Part print with two shaded views. Sizes in mm from the minimum x, y, z corner. Give positions to 0.01 mm unless a question says otherwise; leave off trailing zeros. Write each loop counter-clockwise with the first axis right and the second up, starting at its lowest first coordinate (ties: lowest second). Pieces come first, ordered by that corner, then holes. Notation, with made-up numbers: (80, 85) - (84, 85) arc R30 ccw to (84, 108) - close; hole circle Ø1 at (-25, 62). An arc over 180 degrees is marked (long way). One line per item, written item: value. Start each with the question number.
(1) Drop flat-ended pins along their axis: P1, Ø2, axis at x = 14, z = 26, coming from the -Y side; P2, Ø1.6, axis at x = 95.5, y = 1, coming from the +Z side; P3, Ø1.2, axis at x = 96, y = 1, coming from the -Z side; P4, Ø0.8, axis at x = 7, y = 1, coming from the +Z side (1 decimal). Give the stop position or say it passes through.
(2) Probe L1, parallel to X at y = 2.95, z = 54; L2, parallel to Y at x = 19.5, z = 93.5; L3, parallel to Z at x = 11, y = 1.4 (1 decimal). List the from-to ranges inside material, lowest first.
(3) Cut at A-A, the plane x = 72.5. List the corners of the cut face in (y, z).
(4) Cut at B-B, the plane y = 2.8. List the corners of the cut face in (x, z).
(5) Mould opens along X. For the marked faces 1 and 2 say: pulls with the +X half, pulls with the -X half, needs draft (parallel to the pull), parting line crosses it, or undercut.
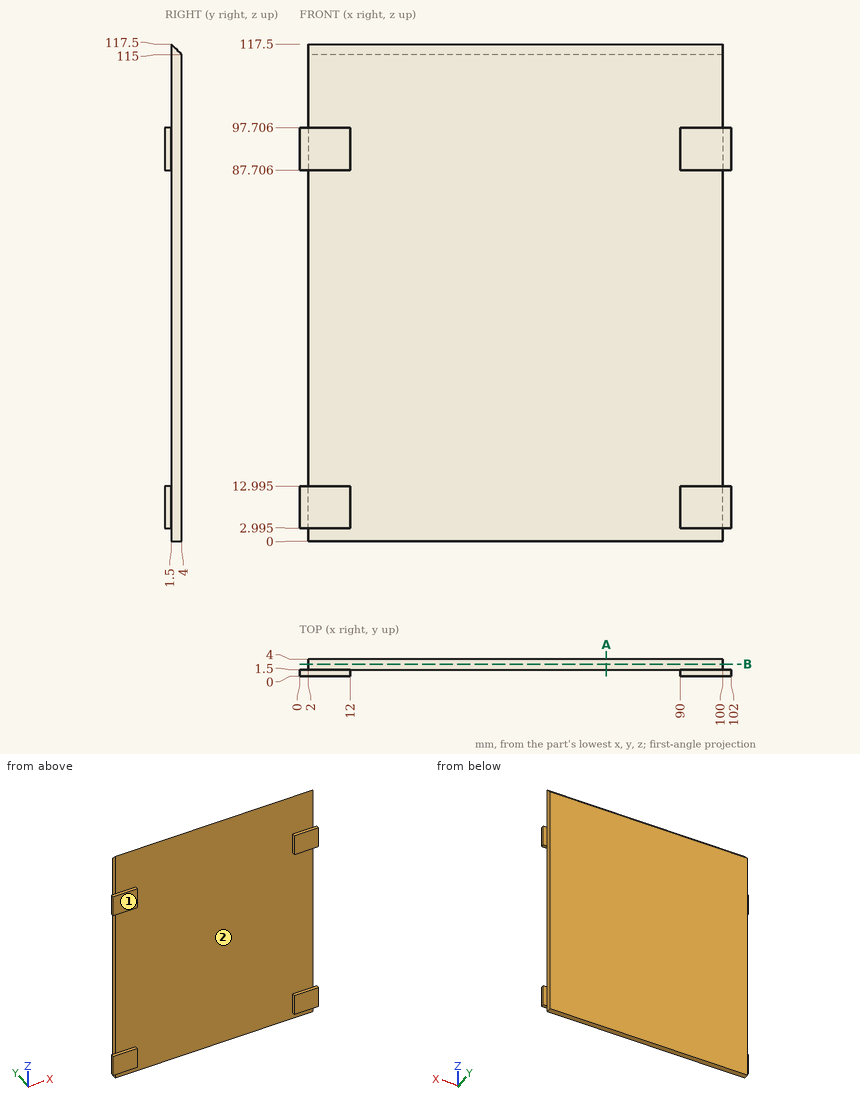
Answers follow:
1. P1: stops at y = 1.5
1. P2: stops at z = 117.5
1. P3: stops at z = 0
1. P4: stops at z = 97.7
2. L1: x = 2 to 100
2. L2: y = 1.5 to 4
2. L3: z = 3 to 13, 87.7 to 97.7
3. outline: (1.5, 0) - (4, 0) - (4, 115) - (1.5, 117.5) - close
4. outline: (2, 0) - (100, 0) - (100, 116.2) - (2, 116.2) - close
5. face 1: needs draft
5. face 2: undercut
